from build123d import *

# Parameters (mm, degrees)
BOSS_EXTRUDE1_DEPTH = 37
BOSS_EXTRUDE2_DEPTH = 2
BOSS_EXTRUDE3_START = -35
BOSS_EXTRUDE3_DEPTH = 2
CUT_EXTRUDE2_DEPTH  = 2
SKETCH8_W           = 15
SKETCH8_H           = 6
SKETCH8_W_2         = 12
SKETCH8_H_2         = 3
CUT_EXTRUDE3_DEPTH  = 10
SKETCH3_R           = 12
CUT_EXTRUDE4_DEPTH  = 10


with BuildPart() as part:
    # Sketch2 → Boss-Extrude1 (new body)
    with BuildSketch(Plane.XY):
        Polygon((0, 0), (7, 0), (7, -20), (34.5, -20), (34.5, 0), (41.5, 0), (41.5, -2), (36.5, -2), (36.5, -22), (5, -22), (5, -2), (0, -2), align=None)
    extrude(amount=BOSS_EXTRUDE1_DEPTH)

    # Sketch5 → Boss-Extrude2 (add)
    with BuildSketch(Plane.XY.offset(37)):
        Polygon((0, 0), (41.5, 0), (41.5, -2), (36.5, -2), (36.5, -22), (5, -22), (5, -2), (0, -2), align=None)
    extrude(amount=BOSS_EXTRUDE2_DEPTH)

    # Sketch5_2 → Boss-Extrude3 (add)
    with BuildSketch(Plane.XY.offset(37).offset(BOSS_EXTRUDE3_START)):
        Polygon((0, 0), (41.5, 0), (41.5, -2), (36.5, -2), (36.5, -22), (5, -22), (5, -2), (0, -2), align=None)
    extrude(amount=-BOSS_EXTRUDE3_DEPTH)

    # Sketch6 → Cut-Extrude2 (cut)
    with BuildSketch(Plane(origin=(0, 0, 0), x_dir=(-1, 0, 0), z_dir=(0, 0, -1))):
        Polygon((-20.75, -9), (-14.75, -9), (-14.75, -6), (-26.75, -6), (-26.75, -9), align=None)
    extrude(amount=-CUT_EXTRUDE2_DEPTH, mode=Mode.SUBTRACT)

    # Sketch8 → Cut-Extrude3 (cut)
    with BuildSketch(Plane(origin=(0, 0, 0), x_dir=(-1, 0, 0), z_dir=(0, 0, -1))):
        with Locations((-20.75, -7.5)):
            Rectangle(SKETCH8_W, SKETCH8_H)
        with Locations((-20.75, -7.5)):
            Rectangle(SKETCH8_W_2, SKETCH8_H_2, mode=Mode.SUBTRACT)
    extrude(amount=-CUT_EXTRUDE3_DEPTH, mode=Mode.SUBTRACT)

    # Sketch3 → Cut-Extrude4 (cut)
    with BuildSketch(Plane.XZ.offset(22)):
        with Locations(Location((20.75, 18.5, 0), (0, 0, 270))):
            Circle(SKETCH3_R)
    extrude(amount=-CUT_EXTRUDE4_DEPTH, mode=Mode.SUBTRACT)


solid = part.part
Model file for the job. Use its own axes, mm. A direction names the side the tool comes from. Coordinates: 2 decimals unless noted, no trailing zeros. Order: outer loops, then holes, each group sorted by start corner. A loop starts at its lowest first (then second) coordinate and runs counter-clockwise, first axis right, second up. Notation, with made-up numbers: M 43.25,-28.5 L 71.25,-28.5 A26 ccw 71.25,5.5 Z; hole C -23.5,42 d8. An arc over 180 degrees is marked long. Return JSON: item names as keys, results as strings.
1. Saw through at D-D (y = -5.25). Give the cut face in (x, z), and give its area (3 significant figures).
Ans:
{"outline": "M 5,0 L 13.25,0 L 13.25,2 L 7,2 L 7,37 L 34.5,37 L 34.5,2 L 28.25,2 L 28.25,0 L 36.5,0 L 36.5,39 L 5,39 Z", "area": "236 mm^2"}
2. Saw through at C-C (y = -17.25). Give the cut face in (x, z), and give its area (3 significant figures).
Ans:
{"outline": "M 5,0 L 36.5,0 L 36.5,39 L 5,39 Z; hole M 7,2 L 34.5,2 L 34.5,37 L 7,37 Z", "area": "266 mm^2"}
3. Saw through at B-B (z = 18.5). Give the cut face in (x, y), and give its area (3 significant figures).
Ans:
{"outline": "M 0,-2 L 5,-2 L 5,-22 L 8.75,-22 L 8.75,-20 L 7,-20 L 7,0 L 0,0 Z; M 32.75,-22 L 36.5,-22 L 36.5,-2 L 41.5,-2 L 41.5,0 L 34.5,0 L 34.5,-20 L 32.75,-20 Z", "area": "115 mm^2"}
4. Tool access for faces 4 (the face through (5, -12, 19)), 5 (the face through (21, -11, 0)), 6 (the face through (39, -2, 19)), 7 (the face through (28.25, -8, 1)), 8 (the face through (7, -10, 19)): list every direction of +Z, -Z, +X, -X, +Y, -Y with a clear straight run to the whole face (end or side of a thin tool).
Ans:
{"face 4": "+Z, -Z, -X, -Y", "face 5": "-Z, +X, -X, +Y, -Y", "face 6": "+Z, -Z, +X, -Y", "face 7": "-Z", "face 8": "+Y"}
5. Saw through at A-A (x = 20.75). Give the cut face in (y, z), and give its area (3 significant figures).
Ans:
{"outline": "M -22,0 L -10.5,0 L -10.5,2 L -20,2 L -20,6.5 L -22,6.5 Z; M -22,30.5 L -20,30.5 L -20,37 L 0,37 L 0,39 L -22,39 Z; M -4.5,0 L 0,0 L 0,2 L -4.5,2 Z", "area": "98.0 mm^2"}
6. Pull direction X, two halves, no side cores. Call faces 1 (the face through (36.5, -12, 19)), 2 (the face through (21, -11, 39)), 3 (the face through (21, -10.5, 1)): +X half, -X half, draft (parallel to the pull), parting line (faces both ways), or undercut.
Ans:
{"face 1": "+X half", "face 2": "draft", "face 3": "undercut"}
7. Drill centre lines: probe 1 along X at (y, z) = (-21.6, 18.5); probe 2 along Z at (x, y) = (9.5, -7); probe 3 along X at (y, z) = (-18.75, 30). Where is each one in solid material? Low to high.
Ans:
{"probe 1": "5 to 8.75, 32.75 to 36.5", "probe 2": "0 to 2, 37 to 39", "probe 3": "5 to 7, 34.5 to 36.5"}
8. Flat gauge pins, fed straight in: pin 1 (6 mm diameter, centred on y = -14, z = 18, fed in from -X); pin 2 (5.5 mm diameter, centred on x = 2.5, z = 21, fed in from -Y); pin 3 (0.6 mm diameter, centred on y = -9, z = 1, fed in from +X); pin 4 (14 mm diameter, centred on x = 26.5, z = 16.5, fed in from +Y). Where does each tip first touch, or does it go through?
Ans:
{"pin 1": "x = 5", "pin 2": "y = -22", "pin 3": "x = 36.5", "pin 4": "y = -20"}
